Autodesk Inventor part; units mm, degrees
ref_plane "YZ Plane" through (0, 0, 0) normal (1, 0, 0) x (0, 1, 0)
ref_plane "XZ Plane" through (0, 0, 0) normal (0, 1, 0) x (-1, 0, 0)
ref_plane "XY Plane" through (0, 0, 0) normal (0, 0, 1) x (1, 0, 0)
sketch "Sketch1" plane through (0, 0, 0) normal (0, 1, 0) x (-1, 0, 0)
  line L0 (0, 0) -> (-50.8, 0)
  line L1 (0, 0) -> (50.8, 0) construction
  line L2 (-25.4, 0) -> (-25.4, 12.7)
  line L3 (-25.4, 0) -> (-12.7, 0) construction
  circle A0 centre (-25.4, 12.7) radius 3.175
  line L4 (-25.4, 12.7) -> (-25.4, 63.5)
  circle A1 centre (-25.4, 63.5) radius 3.175
  line L5 (-50.8, 0) -> (-50.8, 76.2)
  line L6 (-50.8, 0) -> (25.4, 0) construction
  line L7 (0, 0) -> (76.2, 76.2)
  line L8 (0, 0) -> (107.7631, 0) construction
  line L9 (76.2, 76.2) -> (-50.8, 76.2)
  line L10 (76.2, 76.2) -> (58.2395, 58.2395)
  line L11 (76.2, 76.2) -> (101.6, 76.2) construction
  line L12 (58.2395, 58.2395) -> (40.279, 76.2)
  line L13 (49.2592, 67.2197) -> (40.279, 58.2395)
  line L14 (49.2592, 67.2197) -> (61.9592, 67.2197) construction
  line L15 (40.279, 58.2395) -> (22.3185, 40.279)
  circle A2 centre (22.3185, 40.279) radius 3.175
  circle A3 centre (40.279, 58.2395) radius 3.175
  dimension "d0" = 50.8
  dimension "d1" = 180
  dimension "d2" = 12.7
  dimension "d3" = 90
  dimension "d4" = 6.35
  dimension "d5" = 50.8
  dimension "d6" = 6.35
  dimension "d7" = 76.2
  dimension "d8" = 90
  dimension "d9" = 45
  dimension "d10" = 25.4
  dimension "d11" = 135
  dimension "d12" = 12.7
  dimension "d13" = 135
  dimension "d14" = 25.4
  dimension "d15" = 180
  dimension "d16" = 6.35
  dimension "d17" = 6.35
extrude "Extrusion1" add sketch "Sketch1" along normal blind 3.175 contours L0 L5 L9 L12 L7
properties part number "SideGusset"
Verification items for the finished model (mm, model axes). Give positions to 0.01 mm unless a question says otherwise; leave off trailing zeros. Loops run counter-clockwise (first coordinate to the right, second up) from the corner with the lowest first, then second, coordinate; pieces in that order, holes last. Notation, with made-up numbers: M 74.25,39.25 L 117.25,39.25 A12 ccw 117.25,49.25 Z; hole C 40,71.25 d7. An arc over 180 degrees is marked long. One line per question, with ' | ' between items.
Item 1: Depth check by flat-ended pin: P1, Ø4, axis at x = -22.32, z = 40.28, coming from the +Y side. Enter the tip coordinate at first touch or a pass-through.
Completed:
P1: passes through
Item 2: Draft check along X on faces 1 (the face through (-49.385, 1.565, 67.094)), 2 (the face through (-41.74, 1.57, 61.06)), 3 (the face through (9, 0, 39)). Enter one of: +X half, -X half, draft (parallel to the pull), parting line (faces both ways), or undercut.
Completed:
face 1: -X half | face 2: undercut | face 3: draft
Item 3: Section check A-A, the plane x = 25.4. Record the cut outline in (y, z) (3 decimals), plus the area to 3 significant figures.
Completed:
outline: M 0,0 L 3.175,0 L 3.175,9.525 L 0,9.525 Z; M 0,15.875 L 3.175,15.875 L 3.175,60.325 L 0,60.325 Z; M 0,66.675 L 3.175,66.675 L 3.175,76.2 L 0,76.2 Z | area: 202 mm^2
Item 4: Section check B-B, the plane z = 12.7. Record the cut outline in (x, y) (3 decimals).
Completed:
outline: M -12.7,0 L 22.225,0 L 22.225,3.175 L -12.7,3.175 Z; M 28.575,0 L 50.8,0 L 50.8,3.175 L 28.575,3.175 Z
Item 5: Section check D-D, the plane x = -38.5. Record the cut outline in (y, z) (3 decimals).
Completed:
outline: M 0,38.5 L 3.175,38.5 L 3.175,55.61 L 0,55.61 Z; M 0,60.869 L 3.175,60.869 L 3.175,76.2 L 0,76.2 Z
Item 6: Thickness scan on line 1 (Z direction, x = 25.4, y = 1.85) (3 decimals); line 2 (X direction, y = 0.15, z = 42); line 3 (X direction, y = 2.15, z = 63.5) (3 decimals). Record the ranges inside material, lowest first. Write a range as [from, to].
Completed:
line 1: z = [0, 9.525], [15.875, 60.325], [66.675, 76.2] | line 2: x = [-42, -24.99], [-19.65, 50.8] | line 3: x = [-52.979, 22.225], [28.575, 50.8]
Item 7: Section check C-C, the plane y = 1.15. State how many separate pieces and enclosed holes the cut face has, plus the area to 3 significant figures.
Completed:
separate pieces: 1 | enclosed holes: 4 | area: 6,320 mm^2
